```python
from build123d import *

# Parameters (mm, degrees)
SKETCH1_W           = 16
SKETCH1_H           = 16
SKETCH1_W_2         = 10
SKETCH1_H_2         = 10
BOSS_EXTRUDE1_DEPTH = 2
SKETCH2_W           = 12
SKETCH2_H           = 12
SKETCH2_W_2         = 10
SKETCH2_H_2         = 10
BOSS_EXTRUDE2_DEPTH = 7
BOSS_EXTRUDE3_DEPTH = 12
FILLET1_R           = 1


with BuildPart() as part:
    # Sketch1 → Boss-Extrude1 (new body)
    with BuildSketch(Plane.XY):
        Rectangle(SKETCH1_W, SKETCH1_H)
        Rectangle(SKETCH1_W_2, SKETCH1_H_2, mode=Mode.SUBTRACT)
    extrude(amount=BOSS_EXTRUDE1_DEPTH)

    # Sketch2 → Boss-Extrude2 (add)
    with BuildSketch(Plane.XY):
        Rectangle(SKETCH2_W, SKETCH2_H)
        Rectangle(SKETCH2_W_2, SKETCH2_H_2, mode=Mode.SUBTRACT)
    extrude(amount=-BOSS_EXTRUDE2_DEPTH)

    # Sketch3 → Boss-Extrude3 (add)
    with BuildSketch(Plane(origin=(0, 6, 0), x_dir=(1, 0, 0), z_dir=(0, 1, 0))):
        with BuildLine():
            Line((-6, 7), (-6, 6.249625002))
            ThreePointArc((-6, 6.249625002), (-6.851829776, 5.866467368), (-7.200624902, 5))
            Line((-7.200624902, 5), (-7.200624902, 2.5))
            Line((-7.200624902, 2.5), (-7.950624902, 2.5))
            Line((-7.950624902, 2.5), (-7.950624902, 5))
            ThreePointArc((-7.950624902, 5), (-7.382224013, 6.396865912), (-6, 7))
        make_face()
    boss_extrude3 = extrude(amount=-BOSS_EXTRUDE3_DEPTH)

    # Mirror1: Boss-Extrude3 across plane
    add(boss_extrude3.mirror(Plane(origin=(0, 0, 0), x_dir=(0, 0, 1), z_dir=(1, 0, 0))))

    # Fillet1
    fillet1_edges = [part.edges().sort_by_distance(p)[0] for p in [
        (5, -5, -2.5),
        (5, 5, -2.5),
        (-5, 5, -2.5),
        (-5, -5, -2.5),
        (6, 0, -7),
        (-6, 0, -7),
        (8, -8, 1),
        (-8, -8, 1),
        (-8, 8, 1),
        (8, 8, 1),
    ]]
    fillet(fillet1_edges, radius=FILLET1_R)


solid = part.part
```
For this review, take the finished solid that the model builds, in its own axes (mm). A direction names the side the tool comes from. Coordinates: 2 decimals unless noted, no trailing zeros. Write each loop counter-clockwise with the first axis right and the second up, starting at its lowest first coordinate (ties: lowest second). Pieces come first, ordered by that corner, then holes. Notation, with made-up numbers: (-21, 15) - (-5, 15) arc R23 ccw to (-5, 34) - close; hole circle Ø1 at (36, -31). An arc over 180 degrees is marked (long way). Answer in a Markdown table with one row per item. Add a question column.
Q1. We need section B-B, the plane z = -3. State the section outline as (x, y) points, and give its area (3 significant figures).
Q2. We need section A-A, the plane x = 3. State the section outline as (y, z) points.
Q3. Tool access review of faces 1 (the flat face through (0, 6, -4)), 2 (the flat face through (0, 8, 1)), 3 (the cylindrical face through (7.4, 0.08, -6.38)), 4 (the flat face through (7.201, 0, -4)), 5 (the flat face through (0, 5, -2)): name each direction out of +Z, -Z, +X, -X, +Y, -Y from which nothing blocks a thin tool from reaching the whole face with its end or side.
Q4. Draft analysis for pull direction X (two halves, no side actions). For faces 6 (the cylindrical face through (7.699, -7.715, 1.014)), 7 (the cylindrical face through (-7.4, 0.08, -6.38)), 8 (the flat face through (0, -6, -4)), 9 (the cylindrical face through (6.84, 0.08, -5.88)), state which applies: +X half, -X half, draft (parallel to the pull), parting line (faces both ways), or undercut.
Q5. For P1, Ø4, axis at y = -1, z = -3.5, coming from the +X side; P2, Ø3.5, axis at x = 0.5, z = -3, coming from the -Y side; P3, Ø5, axis at x = -3.5, y = -1, coming from the +Z side; P4, Ø1.5, axis at x = 6.5, z = -2, coming from the +Y side, all flat-tipped, find the tip position at first contact; note any pin that passes through.
Q6. We need section C-C, the plane y = -1.5. State the section outline as (x, z) points.
Q7. We need section D-D, the plane z = 0.75. State the section outline as (x, y) points, and give its area (3 significant figures).
Q8. For probe 1 along X at (y, z) = (-4, -4.25); probe 2 along X at (y, z) = (4.5, -4.25); probe 3 along Y at (x, z) = (-3.5, -6), list the stretches that pass through material, from the lowest coordinate up.
Answer list:
| question | item | result |
|---|---|---|
| 1 | outline | (-7.95, -6) - (-7.2, -6) - (-7.2, 6) - (-7.95, 6) - close; (-6, -6) - (6, -6) - (6, 6) - (-6, 6) - close; (7.2, -6) - (7.95, -6) - (7.95, 6) - (7.2, 6) - close; hole (-5, -4) arc R1 ccw to (-4, -5) - (4, -5) arc R1 ccw to (5, -4) - (5, 4) arc R1 ccw to (4, 5) - (-4, 5) arc R1 ccw to (-5, 4) - close |
| 1 | area | 62.9 mm2 |
| 2 | outline | (-8, 0) - (-6, 0) - (-6, -7) - (-5, -7) - (-5, 2) - (-8, 2) - close; (5, -7) - (6, -7) - (6, 0) - (8, 0) - (8, 2) - (5, 2) - close |
| 3 | face 1 | -Z, +X, -X, +Y |
| 3 | face 2 | +Z, -Z, +X, -X, +Y |
| 3 | face 3 | -Z, +X, +Y, -Y |
| 3 | face 4 | +Y, -Y |
| 3 | face 5 | +Z, -Z |
| 4 | face 6 | +X half |
| 4 | face 7 | -X half |
| 4 | face 8 | draft |
| 4 | face 9 | undercut |
| 5 | P1 | stops at x = 7.95 |
| 5 | P2 | stops at y = -6 |
| 5 | P3 | stops at z = 2 |
| 5 | P4 | stops at y = 6 |
| 6 | outline | (-8, 0) - (-6, 0) - (-6, -6.25) arc R1.25 cw to (-7.2, -5) - (-7.2, -2.5) - (-7.95, -2.5) - (-7.95, -5) arc R2 ccw to (-6, -7) - (-5, -7) - (-5, 2) - (-8, 2) - close; (5, -7) - (6, -7) arc R2 ccw to (7.95, -5) - (7.95, -2.5) - (7.2, -2.5) - (7.2, -5) arc R1.25 cw to (6, -6.25) - (6, 0) - (8, 0) - (8, 2) - (5, 2) - close |
| 7 | outline | (-8, -7) arc R1 ccw to (-7, -8) - (7, -8) arc R1 ccw to (8, -7) - (8, 7) arc R1 ccw to (7, 8) - (-7, 8) arc R1 ccw to (-8, 7) - close; hole (-5, -4) arc R1 ccw to (-4, -5) - (4, -5) arc R1 ccw to (5, -4) - (5, 4) arc R1 ccw to (4, 5) - (-4, 5) arc R1 ccw to (-5, 4) - close |
| 7 | area | 156 mm2 |
| 8 | probe 1 | x = -7.95 to -7.2, -6 to -5, 5 to 6, 7.2 to 7.95 |
| 8 | probe 2 | x = -7.95 to -7.2, -6 to -4.87, 4.87 to 6, 7.2 to 7.95 |
| 8 | probe 3 | y = -6 to -5, 5 to 6 |
